Design review of the part built by this model. Coordinates are the model's own, in mm. A direction names the side the tool comes from. Give positions to 0.01 mm unless a question says otherwise; leave off trailing zeros. Loops run counter-clockwise (first coordinate to the right, second up) from the corner with the lowest first, then second, coordinate; pieces in that order, holes last. Notation, with made-up numbers: M 83,13 L 124,13 A17 cw 124,23 Z; hole C 37.25,71.25 d6. An arc over 180 degrees is marked long. Use CSV: the item, a comma, the result in double quotes.
Autodesk Inventor part; units mm, degrees
ref_plane "Work Plane1" through (0, 3.175, 0) normal (0, 1, 0) x (1, 0, 0)
ref_plane "YZ Plane" through (0, 0, 0) normal (1, 0, 0) x (0, 1, 0)
ref_plane "XZ Plane" through (0, 0, 0) normal (0, 1, 0) x (-1, 0, 0)
sketch "Sketch1" plane through (0, 0, 0) normal (0, 0, 1) x (1, 0, 0)
  line L0 (0, 0) -> (31.75, 0)
  line L1 (31.75, 0) -> (31.75, 6.35)
  line L2 (31.75, 6.35) -> (0, 6.35)
  line L3 (0, 6.35) -> (0, 0)
  point P0 (3.175, 3.175)
  point P1 (28.575, 3.175)
  dimension "d0" = 6.35
  dimension "d1" = 31.75
  dimension "d4" = 3.175
  dimension "d5" = 3.175
  dimension "d6" = 3.175
  dimension "d8" = 3.175
extrude "Extrusion1" add sketch "Sketch1" along normal blind 50.8
sketch "Sketch2" plane through (0, 0, 50.8) normal (0, 0, 1) x (1, 0, 0)
  circle A0 centre (3.175, 3.175) radius 1.5875
  circle A1 centre (28.575, 3.175) radius 1.5875
ref_plane "Work Plane1" through (0, 3.175, 0) normal (0, 1, 0) x (1, 0, 0)
sketch "Sketch3" plane through (0, 3.175, 0) normal (0, 1, 0) x (1, 0, 0)
  line L0 (0, 0) -> (31.75, 0)
  line L1 (0, 0) -> (0, -50.8)
  line L2 (31.75, 0) -> (31.75, -50.8)
  line L3 (31.75, -50.8) -> (0, -50.8)
  line L4 (6.35, -6.35) -> (25.4, -6.35)
  line L5 (25.4, -6.35) -> (25.4, -44.45)
  line L6 (25.4, -44.45) -> (6.35, -44.45)
  line L7 (6.35, -44.45) -> (6.35, -6.35)
  line L8 (25.4, -44.45) -> (6.35, -31.75) construction
  line L9 (25.4, -19.05) -> (6.35, -6.35) construction
  line L10 (6.35, -31.75) -> (25.4, -19.05) construction
  line L11 (22.5381, -44.45) -> (6.35, -33.6579)
  line L12 (25.4, -42.5421) -> (9.2119, -31.75)
  line L13 (9.2119, -31.75) -> (25.4, -20.9579)
  line L14 (6.35, -29.8421) -> (22.5381, -19.05)
  line L15 (22.5381, -19.05) -> (6.35, -8.2579)
  line L16 (25.4, -17.1421) -> (9.2119, -6.35)
  point P0 (25.4, -15.6798)
  point P1 (6.35, -19.8802)
  point P2 (6.35, -8.0598)
  point P3 (10.6245, -6.35)
  point P4 (25.4, -12.2602)
  dimension "d27" = 6.35
  dimension "d28" = 6.35
  dimension "d29" = 6.35
  dimension "d30" = 6.35
  dimension "d31" = 33.69
  dimension "d32" = 67.38
  dimension "d33" = 1.5875
  dimension "d34" = 3.175
  dimension "d35" = 1.5875
  dimension "d36" = 3.175
  dimension "d37" = 1.5875
  dimension "d38" = 3.175
extrude "Extrusion4" cut sketch "Sketch3" along normal mid plane 25.4 contours L4 L5 L16 | L15 L14 L7 | L5 L12 L13 | L11 L6 L7
sketch "Sketch5" plane through (0, 6.35, 0) normal (0, 1, 0) x (1, 0, 0)
  line L0 (0, -50.8) -> (31.75, -50.8)
  line L1 (31.75, 0) -> (31.75, -50.8)
  line L2 (0, 0) -> (31.75, 0)
  line L3 (31.75, 0) -> (31.75, -6.35)
  line L4 (31.75, -6.35) -> (0, -6.35)
  line L5 (0, -6.35) -> (0, 0)
  line L6 (0, -6.35) -> (31.75, -6.35)
  line L7 (31.75, -6.35) -> (31.75, -44.45)
  line L8 (31.75, -44.45) -> (0, -44.45)
  line L9 (0, -44.45) -> (0, -6.35)
  line L10 (31.75, -44.45) -> (0, -44.45)
  line L11 (0, -44.45) -> (0, -50.8)
  line L12 (0, -50.8) -> (31.75, -50.8)
  line L13 (31.75, -50.8) -> (31.75, -44.45)
extrude "Extrusion6" cut sketch "Sketch5" against normal blind 1.5875 contours L9 L4 L1 L8
sketch "Sketch6" plane through (0, 0, 0) normal (0, -1, 0) x (1, 0, 0)
  line L0 (0, 0) -> (0, 50.8)
  line L1 (31.75, 0) -> (31.75, 50.8)
  line L2 (0, 50.8) -> (31.75, 50.8)
  line L3 (31.75, 50.8) -> (31.75, 44.45)
  line L4 (31.75, 44.45) -> (0, 44.45)
  line L5 (0, 44.45) -> (0, 50.8)
  line L6 (31.75, 44.45) -> (0, 44.45)
  line L7 (0, 44.45) -> (0, 6.35)
  line L8 (0, 6.35) -> (31.75, 6.35)
  line L9 (31.75, 6.35) -> (31.75, 44.45)
  line L10 (31.75, 0) -> (0, 0)
  line L11 (0, 0) -> (0, 6.35)
  line L12 (0, 6.35) -> (31.75, 6.35)
  line L13 (31.75, 6.35) -> (31.75, 0)
extrude "Extrusion8" cut sketch "Sketch6" against normal blind 1.5875 contours L0 L4 L1 L8
extrude "Extrusion11" add sketch "Sketch3" along normal mid plane 6.35 contours L0 L2 L3 L1 | L4 L16 L5 L13 L12 L6 L11 L7 L14 L15
fillet "Fillet7" radius 2.3813 12 edges at (25.4, 3.175, 17.1421) (22.5381, 3.175, 19.05) (25.4, 3.175, 20.9579) (25.4, 3.175, 42.5421) (22.5381, 3.175, 44.45) (6.35, 3.175, 44.45) (6.35, 3.175, 33.6579) (9.2119, 3.175, 31.75) (6.35, 3.175, 29.8421) (6.35, 3.175, 8.2579) (9.2119, 3.175, 6.35) (25.4, 3.175, 6.35)
extrude "Extrusion12" cut sketch "Sketch2" against normal blind 12.7
hole "Hole2" at (3.175, 3.175, 0) at (28.575, 3.175, 0) direction (0, 0, 1) diameter 3.175 depth 12.7 tip angle 118
thread "Thread5"
thread "Thread6"
thread "Thread7"
thread "Thread8"
equation "\"d28\" = d30"
equation "\"d29\" = d27"
equation "\"d30\" = d29"
equation "\"d32\" = 2 * d31"
equation "\"d34\" = 2 * d33"
equation "\"d35\" = d33"
equation "\"d36\" = d34"
equation "\"d37\" = d35"
equation "\"d38\" = d36"
properties part number "upper gearbox stand off standard"
(1) We need section A-A on y = 0.75. State the section outline as (x, z) points, then the cut area to 3 significant figures.
A:
outline,"M 0,0 L 31.75,0 L 31.75,50.8 L 0,50.8 Z; hole M 6.35,12.71 A2.38 ccw 10.05,10.73 L 19.57,17.07 A2.38 ccw 19.57,21.03 L 10.05,27.37 A2.38 ccw 6.35,25.39 Z; hole M 6.35,38.11 A2.38 ccw 10.05,36.13 L 15.99,40.09 A2.38 ccw 14.67,44.45 L 8.73,44.45 A2.38 ccw 6.35,42.07 Z; hole M 12.18,29.77 L 21.7,23.43 A2.38 ccw 25.4,25.41 L 25.4,38.09 A2.38 ccw 21.7,40.07 L 12.18,33.73 A2.38 ccw Z; hole M 15.76,10.71 A2.38 ccw 17.08,6.35 L 23.02,6.35 A2.38 ccw 25.4,8.73 L 25.4,12.69 A2.38 ccw 21.7,14.67 Z"
area,"1,150 mm²"
(2) We need section D-D on x = 16.5. State the section outline as (y, z) points, then the cut area to 3 significant figures.
A:
outline,"M 0,0 L 6.35,0 L 6.35,6.42 L 0,6.42 Z; M 0,11.21 L 6.35,11.21 L 6.35,15.02 L 0,15.02 Z; M 0,23.08 L 6.35,23.08 L 6.35,26.89 L 0,26.89 Z; M 0,36.61 L 6.35,36.61 L 6.35,40.54 L 0,40.54 Z; M 0,43.6 L 6.35,43.6 L 6.35,50.8 L 0,50.8 Z"
area,"160 mm²"
(3) The part is to be moulded in two halves that separate along Y. For faces 1 (the flat face through (16, 0, 25)), 2 (the flat face through (29, 3, 38.1)), 3 (the flat face through (14.876, 3.131, 13.942)), say which applies: released by +Y, released by -Y, zero draft, split by the parting line, or undercut.
A:
face 1,"released by -Y"
face 2,"undercut"
face 3,"zero draft"
(4) Wall thickness on line 1 along Z through (x, y) = (8.5, 1.25); line 2 along Z through (x, y) = (23, 0.75); line 3 along Z through (x, y) = (20, 4): over which ranges is each line inside the solid? List them lowest first. Write a range as [from, to].
A:
line 1,"[0, 10.34], [27.76, 35.74], [44.44, 50.8]"
line 2,"[0, 6.35], [15.07, 23.03], [40.47, 50.8]"
line 3,"[0, 6.35], [13.54, 17.44], [20.66, 24.56], [38.94, 50.8]"
(5) We need section B-B on z = 39. Count the separate pieces of the cut face and the enclosed holes in it, then the cut area to 3 significant figures.
A:
separate pieces,"3"
enclosed holes,"2"
area,"102 mm²"
(6) Machinability: for faces 4 (the flat face through (0, 3, 25)), 5 (the flat face through (25.4, 3, 11)), 6 (the cylindrical face through (4.141, 1.915, 6.439)), which of the approach directions +Z, -Z, +X, -X, +Y, -Y give a long, thin tool a straight path to every point of the face, cutting with its end or side? Answer none if there is none.
A:
face 4,"+Z, -Z, -X, +Y, -Y"
face 5,"+Y, -Y"
face 6,"-Z"
(7) We need section C-C on z = 16. State the section outline as (x, y) points, then the cut area to 3 significant figures.
A:
outline,"M 0,0 L 6.35,0 L 6.35,6.35 L 0,6.35 Z; M 17.96,0 L 31.75,0 L 31.75,6.35 L 17.96,6.35 Z"
area,"128 mm²"
(8) Clearance check with flat-ended pins moving along their axes: P1, Ø1, axis at x = 28.5, y = 3.5, coming from the +Z side; P2, Ø2.5, axis at x = 3.175, y = 3.175, coming from the -Z side. State where each tip first meets the part, or that it passes through.
A:
P1,"z = 38.1"
P2,"z = 12.9"
